Can you work these out from the drawing? Everything is in mm from the part's minimum corner. Give positions to 0.01 mm unless a question says otherwise; leave off trailing zeros. Write each loop counter-clockwise with the first axis right and the second up, starting at its lowest first coordinate (ties: lowest second). Pieces come first, ordered by that corner, then holes. Notation, with made-up numbers: (-7.5, 13) -> (11.5, 13) arc R16 ccw to (11.5, 24) -> close; hole circle Ø4 at (51, 14.5). An arc over 180 degrees is marked (long way). Use one line per item in the form item = value.
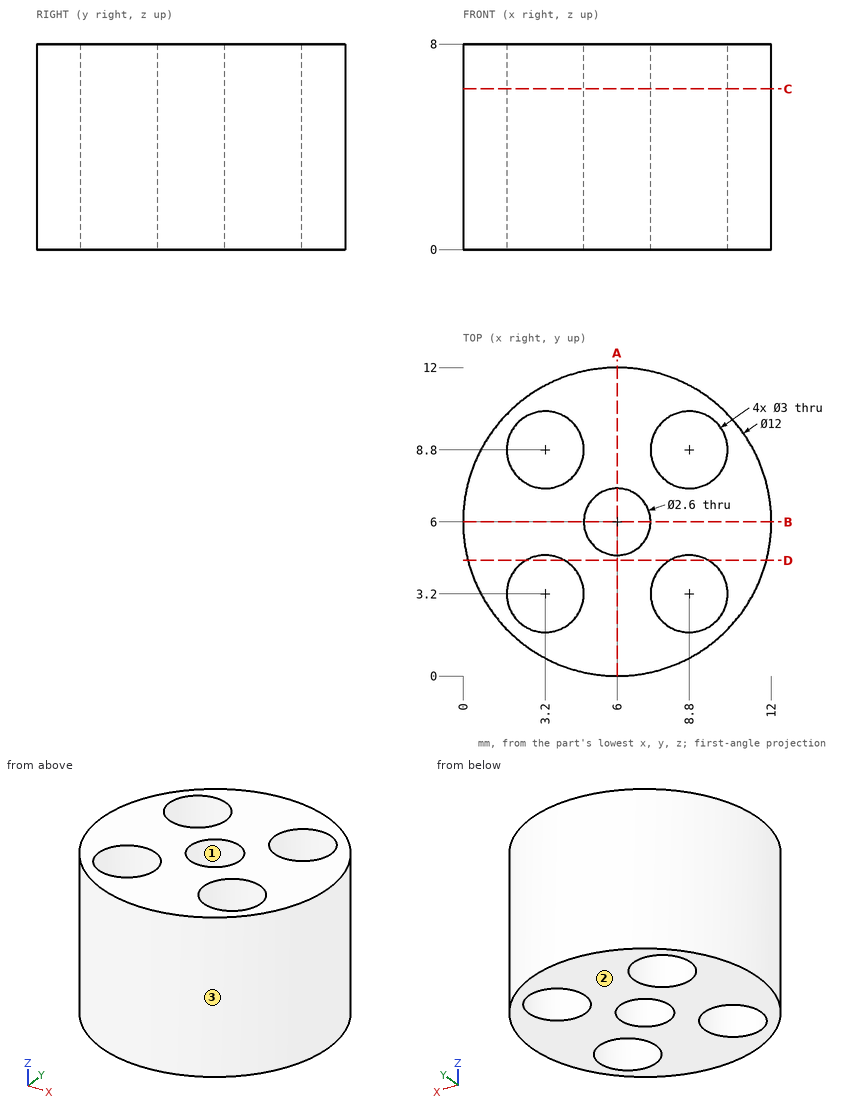
Q1. I want a section at D-D, the plane y = 4.5. Write out the boundary of the cut face in (x, z), and give its area (3 significant figures).
Result set:
outline = (0.19, 0) -> (2.45, 0) -> (2.45, 8) -> (0.19, 8) -> close; (3.95, 0) -> (8.05, 0) -> (8.05, 8) -> (3.95, 8) -> close; (9.55, 0) -> (11.81, 0) -> (11.81, 8) -> (9.55, 8) -> close
area = 69.0 mm2
Q2. If I drill on line 1 along Y through (x, z) = (8.8, 6); line 2 along X through (y, z) = (2.5, 5.25); line 3 along X through (y, z) = (10, 3.75), over which ranges is the centre line in solid material (lowest first)? Write a range as from..to.
Result set:
line_1 = 0.69..1.7, 4.7..7.3, 10.3..11.31
line_2 = 1.13..1.87, 4.53..7.47, 10.13..10.87
line_3 = 1.53..2.3, 4.1..7.9, 9.7..10.47
Q3. I want a section at C-C, the plane z = 6.25. Write out the boundary of the cut face in (x, y), and give its area (3 significant figures).
Result set:
outline = circle Ø12 at (6, 6); hole circle Ø3 at (3.2, 3.2); hole circle Ø3 at (3.2, 8.8); hole circle Ø2.6 at (6, 6); hole circle Ø3 at (8.8, 3.2); hole circle Ø3 at (8.8, 8.8)
area = 79.5 mm2
Q4. I want a section at A-A, the plane x = 6. Write out the boundary of the cut face in (y, z).
Result set:
outline = (0, 0) -> (4.7, 0) -> (4.7, 8) -> (0, 8) -> close; (7.3, 0) -> (12, 0) -> (12, 8) -> (7.3, 8) -> close
Q5. If we mould it in two halves opening along Y, with no side actions, what happens to the marked faces 1, 2 and 3? For each: +Y half, -Y half, draft (parallel to the pull), parting line (faces both ways), or undercut.
Result set:
face_1 = undercut
face_2 = draft
face_3 = parting line
Q6. Will these pins go through, and if not, where does the flat tip stop? pin 1 Ø2 at (x, z) = (2.5, 1.5) entering from -Y; pin 2 Ø3 at (x, z) = (9.5, 2) entering from +Y; pin 3 Ø3 at (x, z) = (2.5, 1) entering from -Y.
Result set:
pin_1 = 0.55
pin_2 = 11.66
pin_3 = 0.34
